from build123d import *

# Parameters (mm, degrees)
BOSS_EXTRUDE1_DEPTH  = 110
SKETCH5_R            = 1.7
BOSS_EXTRUDE2_DEPTH  = 2
CUT_EXTRUDE2_DEPTH   = 122.768226263
SKETCH7_R            = 1.35
CUT_EXTRUDE3_DEPTH   = 10
SKETCH8_R            = 1.35
CUT_EXTRUDE4_DEPTH   = 18
SKETCH9_R            = 1.35
CUT_EXTRUDE5_DEPTH   = 20
CHAMFER3_SIZE        = 1
CUT_EXTRUDE6_DEPTH   = 30
SKETCH17_R           = 0.8
CUT_EXTRUDE11_DEPTH  = 10
SKETCH19_W           = 6
SKETCH19_H           = 20
CUT_EXTRUDE12_DEPTH  = 2
BOSS_EXTRUDE3_DEPTH  = 5
FILLET1_R            = 1
FILLET1_OF_MIRROR2_R = 1
BOSS_EXTRUDE4_DEPTH  = 6
SKETCH22_W           = 6
SKETCH22_H           = 5.520484943
CUT_EXTRUDE13_DEPTH  = 142.567358074


with BuildPart() as part:
    # Sketch1 → Boss-Extrude1 (new body)
    with BuildSketch(Plane(origin=(0, 0, 0), x_dir=(0, 0, -1), z_dir=(1, 0, 0))):
        with BuildLine():
            Line((-14.176031791, 25.95), (14.176031791, 25.95))
            ThreePointArc((14.176031791, 25.95), (40.126031791, 0), (14.176031791, -25.95))
            Line((14.176031791, -25.95), (-14.176031791, -25.95))
            ThreePointArc((-14.176031791, -25.95), (-40.126031791, 0), (-14.176031791, 25.95))
        make_face()
        with BuildLine():
            ThreePointArc((14.176031791, -24.2), (38.376031791, 0), (14.176031791, 24.2))
            Line((14.176031791, 24.2), (-14.176031791, 24.2))
            ThreePointArc((-14.176031791, 24.2), (-38.376031791, 0), (-14.176031791, -24.2))
            Line((-14.176031791, -24.2), (14.176031791, -24.2))
        make_face(mode=Mode.SUBTRACT)
    extrude(amount=-BOSS_EXTRUDE1_DEPTH)

    # Sketch5 → Boss-Extrude2 (add)
    with BuildSketch(Plane(origin=(0, 0, 0), x_dir=(0, 0, -1), z_dir=(1, 0, 0))):
        with BuildLine():
            Line((14.176031791, 25.95), (-14.176031791, 25.95))
            ThreePointArc((-14.176031791, 25.95), (-40.126031791, 0), (-14.176031791, -25.95))
            Line((-14.176031791, -25.95), (14.176031791, -25.95))
            ThreePointArc((14.176031791, -25.95), (40.126031791, 0), (14.176031791, 25.95))
        make_face()
        with Locations((-14.176031791, 0)):
            Circle(SKETCH5_R, mode=Mode.SUBTRACT)
        with Locations((14.176031791, 0)):
            Circle(SKETCH5_R, mode=Mode.SUBTRACT)
    extrude(amount=BOSS_EXTRUDE2_DEPTH)

    # Sketch6 → Cut-Extrude2 (cut, through all)
    with BuildSketch(Plane(origin=(2, 0, 0), x_dir=(0, 0, -1), z_dir=(1, 0, 0))):
        with BuildLine():
            Line((8.197732319, -3.714456195), (-8.197732319, -3.714456195))
            ThreePointArc((-8.197732319, -3.714456195), (0, -9), (8.197732319, -3.714456195))
        make_face()
        with BuildLine():
            ThreePointArc((-8.197732319, 3.714456195), (-9, 0), (-8.197732319, -3.714456195))
            Line((-8.197732319, -3.714456195), (8.197732319, -3.714456195))
            ThreePointArc((8.197732319, -3.714456195), (8.797147005, -1.900053832), (9, 0))
            ThreePointArc((9, 0), (8.797147005, 1.900053832), (8.197732319, 3.714456195))
            Line((8.197732319, 3.714456195), (-8.197732319, 3.714456195))
        make_face()
        with BuildLine():
            ThreePointArc((8.197732319, 3.714456195), (0, 9), (-8.197732319, 3.714456195))
            Line((-8.197732319, 3.714456195), (8.197732319, 3.714456195))
        make_face()
    extrude(amount=-CUT_EXTRUDE2_DEPTH, mode=Mode.SUBTRACT)

    # Sketch7 → Cut-Extrude3 (cut)
    with BuildSketch(Plane(origin=(0, 25.95, 0), x_dir=(1, 0, 0), z_dir=(0, 1, 0))):
        with Locations(Location((-86.907808055, 0, 0), (0, 0, 270))):
            Circle(SKETCH7_R)
    extrude(amount=-CUT_EXTRUDE3_DEPTH, mode=Mode.SUBTRACT)

    # Sketch8 → Cut-Extrude4 (cut)
    with BuildSketch(Plane(origin=(-81.2, -21.801570971, 13.800859089), x_dir=(0, -0.5348639046580952, -0.8449382246613631), z_dir=(0, -0.8449382246613631, 0.5348639046580952))):
        with Locations(Location((-11.851715909, -5.707808055, 0), (0, 0, 180))):
            Circle(SKETCH8_R)
    extrude(amount=CUT_EXTRUDE4_DEPTH, mode=Mode.SUBTRACT)

    # Sketch9 → Cut-Extrude5 (cut)
    with BuildSketch(Plane(origin=(-81.2, -20.415869871, -18.919341673), x_dir=(0, 0.6797127918842137, -0.7334783708801288), z_dir=(0, -0.7334783708801288, -0.6797127918842137))):
        with Locations(Location((10.288299219, -5.707808055, 0), (0, 0, 180))):
            Circle(SKETCH9_R)
    extrude(amount=CUT_EXTRUDE5_DEPTH, mode=Mode.SUBTRACT)

    # Chamfer3
    chamfer3_edges = [part.edges().sort_by_distance(p)[0] for p in [
        (0, -3.714456195, 8.197732319),
    ]]
    chamfer(chamfer3_edges, length=CHAMFER3_SIZE)

    # Sketch11 → Cut-Extrude6 (cut)
    with BuildSketch(Plane.ZY.offset(110)):
        with BuildLine():
            Line((34.47, 13.05), (34.47, 12.05))
            Line((34.47, 12.05), (35.16263466, 12.05))
            ThreePointArc((35.16263466, 12.05), (34.865291248, 12.553666521), (34.555862506, 13.05))
            Line((34.555862506, 13.05), (34.47, 13.05))
        make_face()
        with BuildLine():
            ThreePointArc((34.555862506, 13.05), (34.865291248, 12.553666521), (35.16263466, 12.05))
            Line((35.16263466, 12.05), (35.47, 12.05))
            Line((35.47, 12.05), (35.47, 13.05))
            Line((35.47, 13.05), (34.555862506, 13.05))
        make_face()
        with BuildLine():
            Line((35.47, 12.05), (35.16263466, 12.05))
            ThreePointArc((35.16263466, 12.05), (35.318118105, 11.775066296), (35.47, 11.498126712))
            Line((35.47, 11.498126712), (35.47, 12.05))
        make_face()
        with BuildLine():
            Line((35.16263466, 12.05), (34.47, 12.05))
            Line((34.47, 12.05), (34.47, 10.910793812))
            Line((34.47, 10.910793812), (35.47, 10.910793812))
            Line((35.47, 10.910793812), (35.47, 11.498126712))
            ThreePointArc((35.47, 11.498126712), (35.318118105, 11.775066296), (35.16263466, 12.05))
        make_face()
    extrude(amount=-CUT_EXTRUDE6_DEPTH, mode=Mode.SUBTRACT)

    # Sketch17 → Cut-Extrude11 (cut)
    with BuildSketch(Plane(origin=(0, 25.95, 0), x_dir=(1, 0, 0), z_dir=(0, 1, 0))):
        with Locations(Location((-17.658223223, 13.95, 0), (0, 0, 16.411842871))):
            Circle(SKETCH17_R)
        with Locations(Location((-17.658223223, -13.95, 0), (0, 0, 196.411842871))):
            Circle(SKETCH17_R)
        with Locations(Location((-69.758223223, -19.05, 0), (0, 0, 270))):
            Circle(SKETCH17_R)
    extrude(amount=-CUT_EXTRUDE11_DEPTH, mode=Mode.SUBTRACT)

    # Sketch19 → Cut-Extrude12 (cut)
    with BuildSketch(Plane(origin=(0, 0, -40.126031791), x_dir=(-1, 0, 0), z_dir=(0, 0, -1))):
        with Locations((6, 0)):
            Rectangle(SKETCH19_W, SKETCH19_H)
    cut_extrude12 = extrude(amount=-CUT_EXTRUDE12_DEPTH, mode=Mode.SUBTRACT)

    # Mirror1: Cut-Extrude12 across plane
    add(cut_extrude12.mirror(Plane.XY), mode=Mode.SUBTRACT)

    # Sketch20 → Boss-Extrude3 (add)
    with BuildSketch(Plane.ZY.offset(3)):
        with BuildLine():
            Line((-46.126031791, -4.010005005), (-39.814330483, -4.010005005))
            ThreePointArc((-39.814330483, -4.010005005), (-39.939374777, 3.106872735), (-38.126031791, 9.989994995))
            Line((-38.126031791, 9.989994995), (-46.126031791, 9.989994995))
            ThreePointArc((-46.126031791, 9.989994995), (-46.833138572, 9.697101776), (-47.126031791, 8.989994995))
            Line((-47.126031791, 8.989994995), (-47.126031791, -3.010005005))
            ThreePointArc((-47.126031791, -3.010005005), (-46.833138572, -3.717111786), (-46.126031791, -4.010005005))
        make_face()
        with BuildLine():
            ThreePointArc((-45.726031791, -0.469510052), (-43.726031791, 1.530489948), (-41.726031791, -0.469510052))
            ThreePointArc((-41.726031791, -0.469510052), (-43.726031791, -2.469510052), (-45.726031791, -0.469510052))
        make_face(mode=Mode.SUBTRACT)
        with BuildLine():
            ThreePointArc((-45.726031791, 6.030489948), (-43.726031791, 8.030489948), (-41.726031791, 6.030489948))
            ThreePointArc((-41.726031791, 6.030489948), (-43.726031791, 4.030489948), (-45.726031791, 6.030489948))
        make_face(mode=Mode.SUBTRACT)
    boss_extrude3 = extrude(amount=-BOSS_EXTRUDE3_DEPTH)

    # Fillet1
    fillet1_edges = [part.edges().sort_by_distance(p)[0] for p in [
        (2, 9.989994995, -42.126031791),
        (2, -3.717111786, -46.833138572),
        (2, 9.697101776, -46.833138572),
        (2, -4.010005005, -42.970181137),
        (2, 2.989994995, -47.126031791),
    ]]
    fillet(fillet1_edges, radius=FILLET1_R)

    # Mirror2: Boss-Extrude3 across plane
    add(boss_extrude3.mirror(Plane.XY))

    # Fillet1 of Mirror2
    fillet1_of_mirror2_edges = [part.edges().sort_by_distance(p)[0] for p in [
        (2, 9.989994995, 42.126031791),
        (2, -3.717111786, 46.833138572),
        (2, 9.697101776, 46.833138572),
        (2, -4.010005005, 42.970181137),
        (2, 2.989994995, 47.126031791),
    ]]
    fillet(fillet1_of_mirror2_edges, radius=FILLET1_OF_MIRROR2_R)

    # Sketch21 → Boss-Extrude4 (add)
    with BuildSketch(Plane.ZY.offset(3)):
        with BuildLine():
            Line((-39.814330483, -4.010005005), (-38.126031791, -4.010005005))
            Line((-38.126031791, -4.010005005), (-38.126031791, -9.989994995))
            ThreePointArc((-38.126031791, -9.989994995), (-39.149816283, -7.050715433), (-39.814330483, -4.010005005))
        make_face()
        with BuildLine():
            Line((38.126031791, -4.010005005), (38.126031791, -9.989994995))
            ThreePointArc((38.126031791, -9.989994995), (39.149816283, -7.050715433), (39.814330483, -4.010005005))
            Line((39.814330483, -4.010005005), (38.126031791, -4.010005005))
        make_face()
    extrude(amount=BOSS_EXTRUDE4_DEPTH)

    # Sketch22 → Cut-Extrude13 (cut, through all)
    with BuildSketch(Plane(origin=(0, 0, -38.126031791), x_dir=(-1, 0, 0), z_dir=(0, 0, -1))):
        with Locations((6, 6.229752524)):
            Rectangle(SKETCH22_W, SKETCH22_H)
    extrude(amount=-CUT_EXTRUDE13_DEPTH, mode=Mode.SUBTRACT)


solid = part.part
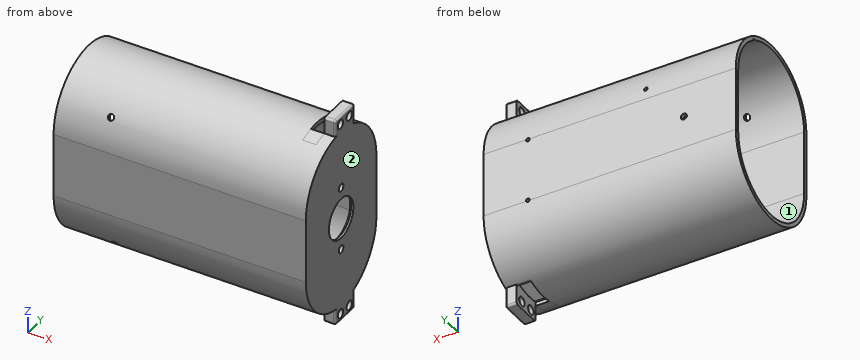
Part model, mm, in its own coordinate system. Face numbers are marked on the shaded views. A direction names the side the tool comes from. Round coordinates to 2 decimals unless told otherwise and drop trailing zeros. Write each loop counter-clockwise with the first axis right and the second up, starting at its lowest first coordinate (ties: lowest second). Pieces come first, ordered by that corner, then holes. Notation, with made-up numbers: (-30, -27.5) - (25, -27.5) arc R21 cw to (25, -23.5) - close; hole circle Ø6 at (7, 78). An arc over 180 degrees is marked (long way). Use CSV: the item, a comma, the result in double quotes.
Item 1: Flat gauge pins, fed straight in: P1, Ø3.5, axis at y = 6.03, z = -43.73, coming from the +X side; P2, Ø2, axis at x = -69.76, z = 19.05, coming from the +Y side; P3, Ø3, axis at y = 4.5, z = 44, coming from the -X side; P4, Ø2, axis at x = -86.91, z = 0, coming from the +Y side. Where does each tip first touch, or does it go through?
Results list:
P1,"passes through"
P2,"stops at y = 25.66"
P3,"stops at x = -3"
P4,"stops at y = -24.2"
Item 2: Slice it at B-B, the plane x = -42.5. Write the cut outline in (y, z).
Results list:
outline,"(-25.95, -14.18) arc R25.95 ccw to (25.95, -14.18) - (25.95, 14.18) arc R25.95 ccw to (-25.95, 14.18) - close; hole (-24.2, -14.18) arc R24.2 ccw to (24.2, -14.18) - (24.2, 14.18) arc R24.2 ccw to (-24.2, 14.18) - close"
Item 3: Slice it at A-A, the plane z = 0. Write the cut outline in (x, y), then the cut area to 3 significant figures.
Results list:
outline,"(-110, -25.95) - (2, -25.95) - (2, -9) - (1, -9) - (0, -10) - (0, -24.2) - (-110, -24.2) - close; (-110, 24.2) - (-88.26, 24.2) - (-88.26, 25.95) - (-110, 25.95) - close; (-85.56, 24.2) - (0, 24.2) - (0, 10) - (1, 9) - (2, 9) - (2, 25.95) - (-85.56, 25.95) - close"
area,"447 mm²"
Item 4: Wall check: L1, parallel to Y at x = -24.5, z = -4; L2, parallel to Y at x = -25.5, z = -25; L3, parallel to Z at x = -23.5, y = -19. Give the ranges that are in metal, low to high.
Results list:
L1,"y = -25.95 to -24.2, 24.2 to 25.95"
L2,"y = -23.58 to -21.64, 21.64 to 23.58"
L3,"z = -31.85 to -29.16, 29.16 to 31.85"
Item 5: Tool access for the marked faces 1 and 2: list every direction of +Z, -Z, +X, -X, +Y, -Y with a clear straight run to the whole face (end or side of a thin tool).
Results list:
face 1,"-X"
face 2,"+Z, -Z, +X, +Y, -Y"
